Check sheet for the drawn part. Datum: minimum x, y, z corner. Units: mm. A direction names the side the tool comes from. Coordinates: 2 decimals unless noted, no trailing zeros. Order: outer loops, then holes, each group sorted by start corner. A loop starts at its lowest first (then second) coordinate and runs counter-clockwise, first axis right, second up. Notation, with made-up numbers: M -18.5,39.25 L -13.5,39.25 A29 ccw -13.5,72.25 Z; hole C 18,-19 d3. An arc over 180 degrees is marked long. Return JSON: item names as keys, results as strings. Group by question number.
Q1. Section check A-A, the plane z = 9. Enter the section's corners in (x, y), then the cut area to 3 significant figures.
Q2. Section check D-D, the plane x = 60. Enter the section's corners in (y, z), then the cut area to 3 significant figures.
Q3. Section check C-C, the plane y = 7.5. Enter the section's corners in (x, z).
Q4. Go/stop test with flat-tipped pins: pin 1 Ø3 at (x, y) = (45.5, 26.5) entering from -Z; pin 2 Ø5 at (x, y) = (34.5, 31) entering from +Z; pin 3 Ø5 at (x, z) = (38, 8.5) entering from -Y. Record where each tip stops, or that it passes through.
Q5. Section check B-B, the plane x = 22.25. Enter the section's corners in (y, z), then the cut area to 3 significant figures.
Q6. Access from +Z, -Z, +X, -X, +Y, -Y to the whole of each face (thin tool, end or side, straight path). Record for the marked faces 1 and 2.
Q7. Thickness scan on probe 1 along Y at (x, z) = (52.25, 2.9); probe 2 along Z at (x, y) = (9, 63); probe 3 along Y at (x, z) = (39.5, 14). Record the ranges inside material, lowest first.
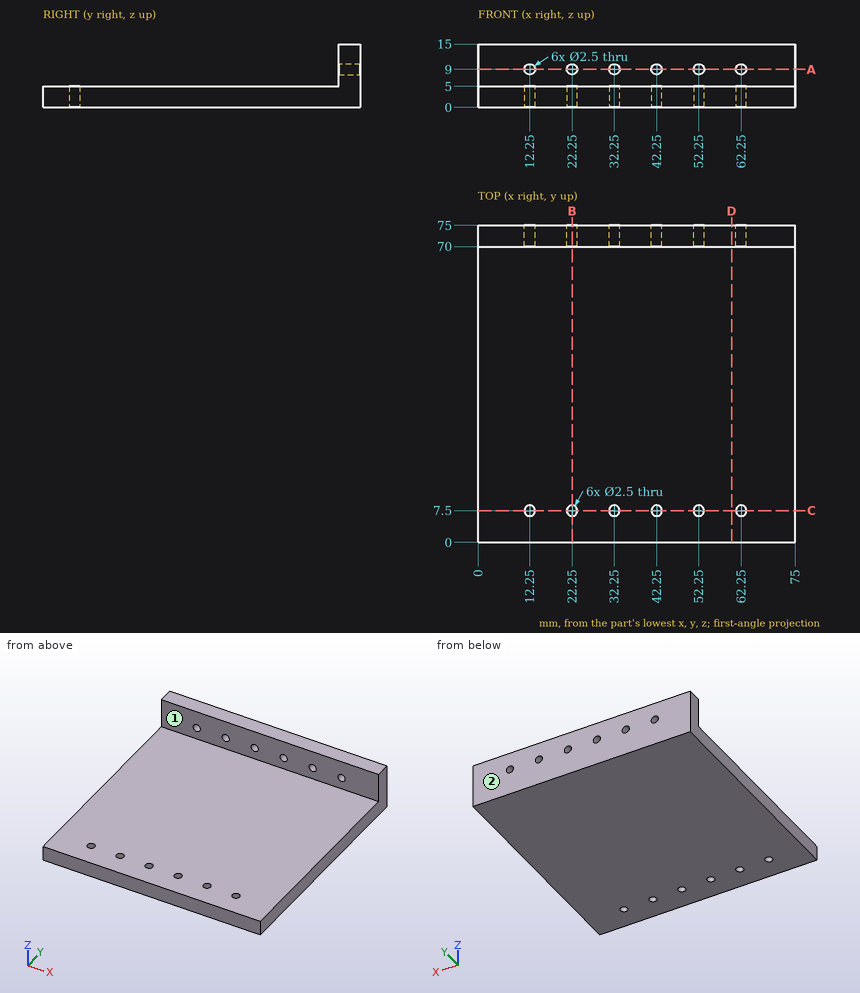
Numbers:
{
 "1": {"outline": "M 0,70 L 11,70 L 11,75 L 0,75 Z; M 13.5,70 L 21,70 L 21,75 L 13.5,75 Z; M 23.5,70 L 31,70 L 31,75 L 23.5,75 Z; M 33.5,70 L 41,70 L 41,75 L 33.5,75 Z; M 43.5,70 L 51,70 L 51,75 L 43.5,75 Z; M 53.5,70 L 61,70 L 61,75 L 53.5,75 Z; M 63.5,70 L 75,70 L 75,75 L 63.5,75 Z", "area": "300 mm2"},
 "2": {"outline": "M 0,0 L 75,0 L 75,15 L 70,15 L 70,5 L 0,5 Z", "area": "425 mm2"},
 "3": {"outline": "M 0,0 L 11,0 L 11,5 L 0,5 Z; M 13.5,0 L 21,0 L 21,5 L 13.5,5 Z; M 23.5,0 L 31,0 L 31,5 L 23.5,5 Z; M 33.5,0 L 41,0 L 41,5 L 33.5,5 Z; M 43.5,0 L 51,0 L 51,5 L 43.5,5 Z; M 53.5,0 L 61,0 L 61,5 L 53.5,5 Z; M 63.5,0 L 75,0 L 75,5 L 63.5,5 Z"},
 "4": {"pin 1": "stops at z = 0", "pin 2": "stops at z = 5", "pin 3": "stops at y = 70"},
 "5": {"outline": "M 0,0 L 6.25,0 L 6.25,5 L 0,5 Z; M 8.75,0 L 75,0 L 75,7.75 L 70,7.75 L 70,5 L 8.75,5 Z; M 70,10.25 L 75,10.25 L 75,15 L 70,15 Z", "area": "400 mm2"},
 "6": {"face 1": "+Z, +X, -X, -Y", "face 2": "+Z, -Z, +X, -X, +Y"},
 "7": {"probe 1": "y = 0 to 6.25, 8.75 to 75", "probe 2": "z = 0 to 5", "probe 3": "y = 70 to 75"}
}
